```python
from build123d import *

# Parameters (mm, degrees)
SKETCH1_W                = 4
SKETCH1_H                = 4
BOSS_EXTRUDE1_DEPTH      = 30
SKETCH2_R                = 2
SKETCH2_R_2              = 1
BOSS_EXTRUDE2_DEPTH      = 4
SKETCH3_R                = 1
CUT_EXTRUDE1_DEPTH       = 33.310988843
BOSS_EXTRUDE3_DEPTH      = 2
BOSS_EXTRUDE3_DEPTH_BACK = 6
SKETCH4_R                = 3.5
SKETCH4_R_2              = 1
SKETCH5_R                = 1
CUT_EXTRUDE2_DEPTH       = 34.170016581
CUT_EXTRUDE3_DEPTH       = 10
CUT_EXTRUDE3_DEPTH_BACK  = 2
SKETCH6_W                = 2
SKETCH6_H                = 5


with BuildPart() as part:
    # Sketch1 → Boss-Extrude1 (new body)
    with BuildSketch(Plane.XY):
        Rectangle(SKETCH1_W, SKETCH1_H)
    extrude(amount=BOSS_EXTRUDE1_DEPTH)

    # Sketch2 → Boss-Extrude2 (add)
    with BuildSketch(Plane(origin=(2, 0, 0), x_dir=(0, 0, -1), z_dir=(1, 0, 0))):
        with Locations((-30, 0)):
            Circle(SKETCH2_R)
        with Locations((-30, 0)):
            Circle(SKETCH2_R_2, mode=Mode.SUBTRACT)
    extrude(amount=-BOSS_EXTRUDE2_DEPTH)

    # Sketch3 → Cut-Extrude1 (cut, through all)
    with BuildSketch(Plane(origin=(2, 0, 0), x_dir=(0, 0, -1), z_dir=(1, 0, 0))):
        with Locations(Location((-30, 0, 0), (0, 0, 90))):
            Circle(SKETCH3_R)
    extrude(amount=-CUT_EXTRUDE1_DEPTH, mode=Mode.SUBTRACT)

    # Sketch4 → Boss-Extrude3 (add, two sides: drawn at the far end of the back side and taken through both)
    with BuildSketch(Plane(origin=(2, 0, 0), x_dir=(0, 0, -1), z_dir=(1, 0, 0)).offset(-BOSS_EXTRUDE3_DEPTH_BACK)):
        with Locations(Location((0, 0, 0), (0, 0, 90))):
            Circle(SKETCH4_R)
        with Locations(Location((0, 0, 0), (0, 0, 90))):
            Circle(SKETCH4_R_2, mode=Mode.SUBTRACT)
    extrude(amount=BOSS_EXTRUDE3_DEPTH + BOSS_EXTRUDE3_DEPTH_BACK)

    # Sketch5 → Cut-Extrude2 (cut, through all)
    with BuildSketch(Plane(origin=(4, 0, 0), x_dir=(0, 0, -1), z_dir=(1, 0, 0))):
        with Locations(Location((0, 0, 0), (0, 0, 90))):
            Circle(SKETCH5_R)
    extrude(amount=-CUT_EXTRUDE2_DEPTH, mode=Mode.SUBTRACT)

    # Sketch6 → Cut-Extrude3 (cut, two sides: drawn at the far end of the back side and taken through both)
    with BuildSketch(Plane.XY.offset(29).offset(-CUT_EXTRUDE3_DEPTH_BACK)):
        Rectangle(SKETCH6_W, SKETCH6_H)
    extrude(amount=CUT_EXTRUDE3_DEPTH + CUT_EXTRUDE3_DEPTH_BACK, mode=Mode.SUBTRACT)


solid = part.part
```
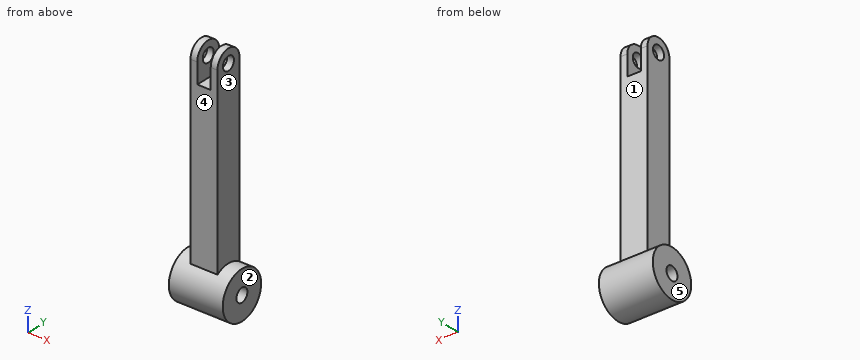
For this review, take the finished solid that the model builds, in its own axes (mm). Face numbers are marked on the shaded views. A direction names the side the tool comes from. Give positions to 0.01 mm unless a question says otherwise; leave off trailing zeros. Write each loop counter-clockwise with the first axis right and the second up, starting at its lowest first coordinate (ties: lowest second). Pieces come first, ordered by that corner, then holes. Notation, with made-up numbers: M 30,83.25 L 62,83.25 A20 cw 62,87.25 Z; hole C 10.25,-33.75 d6. An arc over 180 degrees is marked long. One line per item, written item: value.
1) For the marked faces 1 and 2, list the 3-axis set-ups (+Z, -Z, +X, -X, +Y, -Y) from which the entire face can be reached by the end or side of a thin tool; tool diameter is ignored.
Results are:
face 1: +Z, +X, -X, +Y
face 2: +Z, -Z, +X, +Y, -Y
2) For line 1 (Z direction, x = -1.65, y = 0); line 2 (Z direction, x = 2.25, y = 0); line 3 (Z direction, x = 0, y = 0), list the stretches that pass through material, from the lowest coordinate up. Write a range as from..to.
Results are:
line 1: z = -3.5..-1, 1..29, 31..32
line 2: z = -3.5..-1, 1..3.5
line 3: z = -3.5..-1, 1..27
3) For P1, Ø3, axis at x = 1, z = 12.5, coming from the -Y side; P2, Ø2, axis at y = -0.5, z = 17.5, coming from the +X side; P3, Ø4, axis at x = 1, y = -1.5, coming from the -Z side; P4, Ø4.5, axis at x = 0, z = 13.5, coming from the +Y side, all flat-tipped, find the tip position at first contact; note any pin that passes through.
Results are:
P1: stops at y = -2
P2: stops at x = 2
P3: stops at z = -3.5
P4: stops at y = 2
4) Take a section at A-A, the plane y = 0. Write out the cut boundary in (x, z), then the cut area to 3 significant figures.
Results are:
outline: M -4,-3.5 L 4,-3.5 L 4,-1 L -4,-1 Z; M -4,1 L 4,1 L 4,3.5 L 2,3.5 L 2,29 L 1,29 L 1,27 L -1,27 L -1,29 L -2,29 L -2,3.5 L -4,3.5 Z; M -2,31 L -1,31 L -1,32 L -2,32 Z; M 1,31 L 2,31 L 2,32 L 1,32 Z
area: 140 mm²
5) Take a section at D-D, the plane z = 21. Write out the cut boundary in (x, y).
Results are:
outline: M -2,-2 L 2,-2 L 2,2 L -2,2 Z
6) The part is to be moulded in two halves that separate along X. For the marked faces 3, 4 and 5, say which applies: +X half, -X half, draft (parallel to the pull), parting line (faces both ways), or undercut.
Results are:
face 3: +X half
face 4: draft
face 5: -X half
7) Take a section at B-B, the plane z = 0. Write out the cut boundary in (x, y).
Results are:
outline: M -4,-3.5 L 4,-3.5 L 4,-1 L -4,-1 Z; M -4,1 L 4,1 L 4,3.5 L -4,3.5 Z
8) Take a section at C-C, the plane x = -2.75. Write out the cut boundary in (y, z), then the cut area to 3 significant figures.
Results are:
outline: C 0,0 d7; hole C 0,0 d2
area: 35.3 mm²
